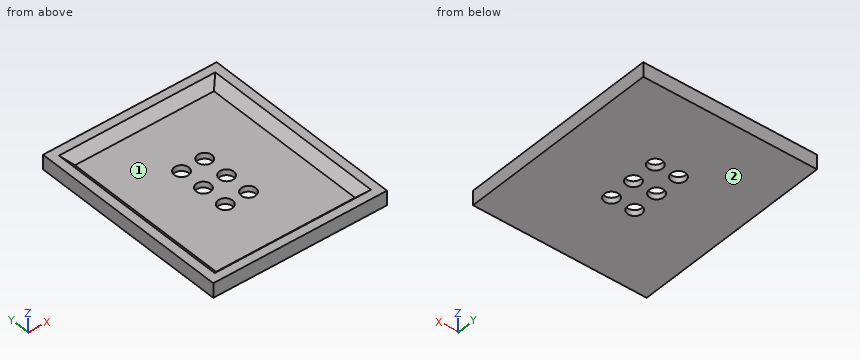
```python
from build123d import *

# Parameters (mm, degrees)
F0_W         = 88.9
F0_H         = 6.35
F1_DEPTH     = 76.2
F2_T         = -2.54
F3_T4_DEPTH  = 83.82
F3_T9_DEPTH  = 71.12
F3_T14_DEPTH = 83.82
F3_T19_DEPTH = 71.12
F5_D         = 6.35
F5_DEPTH     = 12.7
F5_TIP       = 1.9077324654


# Not quite as in the source:
# - a fillet or chamfer that OpenCascade refuses, or shapes differently, is made with other operations: its cross-section is extruded or revolved along the edge and cut away or added


with BuildPart() as f1:
    # F0 (on Right) → F1 (new body)
    with BuildSketch(Plane.YZ):
        with Locations((12.1882097632, -0.3118954591)):
            Rectangle(F0_W, F0_H)
    extrude(amount=F1_DEPTH)

    # F2
    f2_openings = [f1.faces().sort_by_distance(p)[0] for p in [
        (38.1, 12.18821, 2.863105),
    ]]
    offset(amount=F2_T, openings=f2_openings)

    # F3: chamfer of 5.08 on 4 edges, made by hand


with BuildPart() as f3_tool2:
    # F3_s3 → F3_t4 (new body)
    with BuildSketch(Plane.XZ.offset(-54.0982097632)):
        Polygon((2.54, 4.1331045409), (7.62, -0.9468954591), (2.54, -0.9468954591), align=None)
    extrude(amount=F3_T4_DEPTH)

    split(bisect_by=Plane.XY.offset(2.8631045409), keep=Keep.BOTTOM)


with BuildPart() as f1_1:
    add(f1.part)

    # F3_t1: union F3_tool2
    add(f3_tool2.part)


with BuildPart() as f3_tool7:
    # F3_s8 → F3_t9 (new body)
    with BuildSketch(Plane.YZ.offset(2.54)):
        Polygon((-29.7217902368, 4.1331045409), (-24.6417902368, -0.9468954591), (-29.7217902368, -0.9468954591), align=None)
    extrude(amount=F3_T9_DEPTH)

    split(bisect_by=Plane.XY.offset(2.8631045409), keep=Keep.BOTTOM)


with BuildPart() as f1_2:
    add(f1_1.part)

    # F3_t6: union F3_tool7
    add(f3_tool7.part)


with BuildPart() as f3_tool12:
    # F3_s13 → F3_t14 (new body)
    with BuildSketch(Plane.XZ.offset(-54.0982097632)):
        Polygon((73.66, 4.1331045409), (68.58, -0.9468954591), (73.66, -0.9468954591), align=None)
    extrude(amount=F3_T14_DEPTH)

    split(bisect_by=Plane.XY.offset(2.8631045409), keep=Keep.BOTTOM)


with BuildPart() as f1_3:
    add(f1_2.part)

    # F3_t11: union F3_tool12
    add(f3_tool12.part)


with BuildPart() as f3_tool17:
    # F3_s18 → F3_t19 (new body)
    with BuildSketch(Plane.YZ.offset(73.66)):
        Polygon((54.0982097632, 4.1331045409), (49.0182097632, -0.9468954591), (54.0982097632, -0.9468954591), align=None)
    extrude(amount=-F3_T19_DEPTH)

    split(bisect_by=Plane.XY.offset(2.8631045409), keep=Keep.BOTTOM)


with BuildPart() as f1_4:
    add(f1_3.part)

    # F3_t16: union F3_tool17
    add(f3_tool17.part)

    # F5
    with Locations(Plane.XY.offset(-0.9468954591)):
        with Locations((33.02, 23.6182097632), (43.18, 23.6182097632), (43.18, 12.1882097632), (33.02, 12.1882097632), (33.02, 0.7582097632), (43.18, 0.7582097632)):
            Hole(F5_D / 2, depth=F5_DEPTH)
            with Locations((0, 0, -(F5_DEPTH + F5_TIP / 2))):  # 118° drill point
                Cone(0, F5_D / 2, F5_TIP, mode=Mode.SUBTRACT)


solid = f1_4.part
```
CAD build for the part. Positions are in the model's coordinates, mm. Face numbers are marked on the shaded views. Coordinates: 2 decimals unless noted, no trailing zeros. Order: outer loops, then holes, each group sorted by start corner. A loop starts at its lowest first (then second) coordinate and runs counter-clockwise, first axis right, second up. Notation, with made-up numbers: M 29.25,73.25 L 33.25,73.25 A28 cw 33.25,94.25 Z; hole C 56.5,71 d5. An arc over 180 degrees is marked long. Answer as CSV lines item,"result".
1) Mould opens along X. For the marked faces 1 and 2 say: released by +X, released by -X, zero draft, split by the parting line, or undercut.
Verdict:
face 1,"undercut"
face 2,"zero draft"
2) Cut at C-C (z = 0.75). List the corners of the cut face in (x, y), then the cut area to 3 significant figures.
Verdict:
outline,"M 0,-32.26 L 76.2,-32.26 L 76.2,56.64 L 0,56.64 Z; hole M 5.92,-26.34 L 70.28,-26.34 L 70.28,50.72 L 5.92,50.72 Z"
area,"1,820 mm2"
3) Cut at A-A (x = 43.18). List the corners of the cut face in (y, z), then the cut area to 3 significant figures.
Verdict:
outline,"M -32.26,-3.49 L -2.42,-3.49 L -2.42,-0.95 L -24.64,-0.95 L -28.45,2.86 L -32.26,2.86 Z; M 3.93,-3.49 L 9.01,-3.49 L 9.01,-0.95 L 3.93,-0.95 Z; M 15.36,-3.49 L 20.44,-3.49 L 20.44,-0.95 L 15.36,-0.95 Z; M 26.79,-3.49 L 56.64,-3.49 L 56.64,2.86 L 52.83,2.86 L 49.02,-0.95 L 26.79,-0.95 Z"
area,"221 mm2"
4) Flat gauge pins, fed straight in: P1, Ø2, axis at x = 39.5, y = -11.5, coming from the +Z side; P2, Ø4, axis at x = 33.02, y = 23.62, coming from the -Z side. Where does each tip first touch, or does it go through?
Verdict:
P1,"z = -0.95"
P2,"through"
5) Cut at B-B (x = 55). List the corners of the cut face in (y, z).
Verdict:
outline,"M -32.26,-3.49 L 56.64,-3.49 L 56.64,2.86 L 52.83,2.86 L 49.02,-0.95 L -24.64,-0.95 L -28.45,2.86 L -32.26,2.86 Z"
6) Drill centre lines: L1, parallel to Y at x = 43.18, z = -2.05; L2, parallel to X at y = 26, z = -2.25; L3, parallel to X at y = -26, z = 1. Where is each one in solid material? Low to high. Write a range as from..to.
Verdict:
L1,"-32.26..-2.42, 3.93..9.01, 15.36..20.44, 26.79..56.64"
L2,"0..30.92, 35.12..41.08, 45.28..76.2"
L3,"0..5.67, 70.53..76.2"
